```python
from build123d import *

# Parameters (mm, degrees)
BOSS_EXTRUDE1_DEPTH = 88
CUT_EXTRUDE1_DEPTH  = 79
SKETCH4_R           = 7.5
CUT_EXTRUDE2_DEPTH  = 47
SKETCH6_R           = 7.5
CUT_EXTRUDE4_DEPTH  = 47
CUT_EXTRUDE5_START  = -47
SKETCH7_R           = 7.5
CUT_EXTRUDE5_DEPTH  = 47
CUT_EXTRUDE6_START  = -47
SKETCH8_R           = 7.5
CUT_EXTRUDE6_DEPTH  = 47
CUT_EXTRUDE8_DEPTH  = 6


with BuildPart() as part:
    # Sketch1 → Boss-Extrude1 (new body)
    with BuildSketch(Plane(origin=(0, 0, 0), x_dir=(1, 0, 0), z_dir=(0, 1, 0))):
        Polygon((-161.642165003, 149.218305812), (-91.642165003, 149.218305812), (-20.931486885, 78.507627693), (99.068513115, 78.507627693), (169.779191234, 149.218305812), (239.779191234, 149.218305812), (239.779191234, 79.218305812), (169.068513115, 8.507627693), (169.068513115, -111.492372307), (239.779191234, -182.203050426), (239.779191234, -252.203050426), (169.779191234, -252.203050426), (99.068513115, -181.492372307), (-20.931486885, -181.492372307), (-91.642165003, -252.203050426), (-161.642165003, -252.203050426), (-161.642165003, -182.203050426), (-90.931486885, -111.492372307), (-90.931486885, 8.507627693), (-161.642165003, 79.218305812), align=None)
    extrude(amount=BOSS_EXTRUDE1_DEPTH)

    # Sketch3 → Cut-Extrude1 (cut)
    with BuildSketch(Plane(origin=(0, 88, 0), x_dir=(1, 0, 0), z_dir=(0, 1, 0))):
        Polygon((-158.642165003, 146.218305812), (-158.642165003, 80.460946499), (-87.931486885, 9.75026838), (-87.931486885, -112.735012994), (-158.642165003, -183.445691113), (-158.642165003, -249.203050426), (-92.88480569, -249.203050426), (-22.174127572, -178.492372307), (100.311153802, -178.492372307), (171.021831921, -249.203050426), (236.779191234, -249.203050426), (236.779191234, -183.445691113), (166.068513115, -112.735012994), (166.068513115, 9.75026838), (236.779191234, 80.460946499), (236.779191234, 146.218305812), (171.021831921, 146.218305812), (100.311153802, 75.507627693), (-22.174127572, 75.507627693), (-92.88480569, 146.218305812), align=None)
    extrude(amount=-CUT_EXTRUDE1_DEPTH, mode=Mode.SUBTRACT)

    # Sketch4 → Cut-Extrude2 (cut)
    with BuildSketch(Plane(origin=(239.779191234, 0, 0), x_dir=(0, 0, -1), z_dir=(1, 0, 0))):
        with Locations((-207.203050426, 53)):
            Circle(SKETCH4_R)
    extrude(amount=-CUT_EXTRUDE2_DEPTH, mode=Mode.SUBTRACT)

    # Sketch6 → Cut-Extrude4 (cut)
    with BuildSketch(Plane(origin=(239.779191234, 0, 0), x_dir=(0, 0, -1), z_dir=(1, 0, 0))):
        with Locations((104.218305812, 53)):
            Circle(SKETCH6_R)
    extrude(amount=-CUT_EXTRUDE4_DEPTH, mode=Mode.SUBTRACT)

    # Sketch7 → Cut-Extrude5 (cut)
    with BuildSketch(Plane.ZY.offset(161.642165003).offset(CUT_EXTRUDE5_START)):
        with Locations(Location((-104.218305812, 53, 0), (0, 0, 180))):
            Circle(SKETCH7_R)
    extrude(amount=CUT_EXTRUDE5_DEPTH, mode=Mode.SUBTRACT)

    # Sketch8 → Cut-Extrude6 (cut)
    with BuildSketch(Plane.ZY.offset(161.642165003).offset(CUT_EXTRUDE6_START)):
        with Locations(Location((207.203050426, 53, 0), (0, 0, 180))):
            Circle(SKETCH8_R)
    extrude(amount=CUT_EXTRUDE6_DEPTH, mode=Mode.SUBTRACT)

    # Sketch17 → Cut-Extrude8 (cut)
    with BuildSketch(Plane.XZ):
        Polygon((100.311153802, -75.507627693), (171.021831921, -146.218305812), (236.779191234, -146.218305812), (236.779191234, -80.460946499), (166.068513115, -9.75026838), (166.068513115, 112.735012994), (236.779191234, 183.445691113), (236.779191234, 249.203050426), (171.021831921, 249.203050426), (100.311153802, 178.492372307), (-22.174127572, 178.492372307), (-92.88480569, 249.203050426), (-158.642165003, 249.203050426), (-158.642165003, 183.445691113), (-87.931486885, 112.735012994), (-87.931486885, -9.75026838), (-158.642165003, -80.460946499), (-158.642165003, -146.218305812), (-92.88480569, -146.218305812), (-22.174127572, -75.507627693), align=None)
    extrude(amount=-CUT_EXTRUDE8_DEPTH, mode=Mode.SUBTRACT)


solid = part.part
```
Model file for the job. Use its own axes, mm. A direction names the side the tool comes from. Give positions to 0.01 mm unless a question says otherwise; leave off trailing zeros. Loops run counter-clockwise (first coordinate to the right, second up) from the corner with the lowest first, then second, coordinate; pieces in that order, holes last. Notation, with made-up numbers: (86, 14.5) -> (137, 14.5) arc R20 cw to (137, 42.5) -> close; hole circle Ø5 at (6, -19). An arc over 180 degrees is marked (long way). Write each question's results on one line, items separated by ' | '.
(1) Cut at D-D on x = 23.5. List the corners of the cut face in (y, z), and give its area (3 significant figures).
Geometry results:
outline: (0, -78.51) -> (88, -78.51) -> (88, -75.51) -> (9, -75.51) -> (9, 178.49) -> (88, 178.49) -> (88, 181.49) -> (0, 181.49) -> (0, 178.49) -> (6, 178.49) -> (6, -75.51) -> (0, -75.51) -> close | area: 1,290 mm²
(2) Tool access for faces 1 (the flat face through (204.92, 43.38, -44.36)), 2 (the flat face through (166.069, 49, 52)), 3 (the cylindrical face through (-160.121, 55.873, 200.275)), 4 (the flat face through (-125.792, 43.384, -43.368)): list every direction of +Z, -Z, +X, -X, +Y, -Y with a clear straight run to the whole face (end or side of a thin tool).
Geometry results:
face 1: +X, +Y, -Y | face 2: +Y | face 3: -X | face 4: -X, +Y, -Y
(3) Cut at A-A on x = -101. List the corners of the cut face in (y, z), and give its area (3 significant figures).
Geometry results:
outline: (0, -149.22) -> (88, -149.22) -> (88, -146.22) -> (9, -146.22) -> (9, -22.82) -> (88, -22.82) -> (88, -18.58) -> (0, -18.58) -> (0, -22.82) -> (6, -22.82) -> (6, -146.22) -> (0, -146.22) -> close; (0, 121.56) -> (88, 121.56) -> (88, 125.8) -> (9, 125.8) -> (9, 249.2) -> (88, 249.2) -> (88, 252.2) -> (0, 252.2) -> (0, 249.2) -> (6, 249.2) -> (6, 125.8) -> (0, 125.8) -> close | area: 2,020 mm²
(4) Probe line 1 along X through (y, z) = (40.5, 55.5); line 2 along X through (y, z) = (40.5, 219); line 3 along Z through (x, y) = (167.5, 19). List the from-to ranges inside material, lowest first.
Geometry results:
line 1: x = -90.93 to -87.93, 166.07 to 169.07 | line 2: x = -161.64 to -158.64, -62.68 to -58.44, 136.58 to 140.82, 236.78 to 239.78 | line 3: z = -146.94 to -142.7, -11.18 to 114.17, 245.68 to 249.92
(5) Cut at C-C on y = 53. Give the number of separate pieces and of enclosed holes in the cut face, and give its area (3 significant figures).
Geometry results:
separate pieces: 4 | enclosed holes: 0 | area: 5,300 mm²
(6) Flat gauge pins, fed straight in: pin 1 Ø6 at (y, z) = (68, 101) entering from +X; pin 2 Ø9 at (y, z) = (53, 207.2) entering from -X; pin 3 Ø6.5 at (x, y) = (12, 3) entering from -Z. Where does each tip first touch, or does it go through?
Geometry results:
pin 1: stops at x = 169.07 | pin 2: stops at x = -55.38 | pin 3: stops at z = -78.51
(7) Cut at B-B on z = 191. List the corners of the cut face in (x, y).
Geometry results:
outline: (-161.64, 0) -> (-158.64, 0) -> (-158.64, 6) -> (-34.68, 6) -> (-34.68, 0) -> (-30.44, 0) -> (-30.44, 88) -> (-34.68, 88) -> (-34.68, 9) -> (-158.64, 9) -> (-158.64, 88) -> (-161.64, 88) -> close; (108.58, 0) -> (112.82, 0) -> (112.82, 6) -> (236.78, 6) -> (236.78, 0) -> (239.78, 0) -> (239.78, 88) -> (236.78, 88) -> (236.78, 9) -> (112.82, 9) -> (112.82, 88) -> (108.58, 88) -> close
(8) Pull direction Y, two halves, no side cores. Call faces 5 (the cylindrical face through (238.3, 46.346, -107.679)), 6 (the flat face through (36, 6, 54)), 7 (the flat face through (-161.642, 43, 218)): released by +Y, released by -Y, zero draft, split by the parting line, or undercut.
Geometry results:
face 5: undercut | face 6: released by -Y | face 7: zero draft
